Design review of the part built by this model. Coordinates are the model's own, in mm. Face numbers are marked on the shaded views. Give positions to 0.01 mm unless a question says otherwise; leave off trailing zeros. Order: outer loops, then holes, each group sorted by start corner. A loop starts at its lowest first (then second) coordinate and runs counter-clockwise, first axis right, second up.
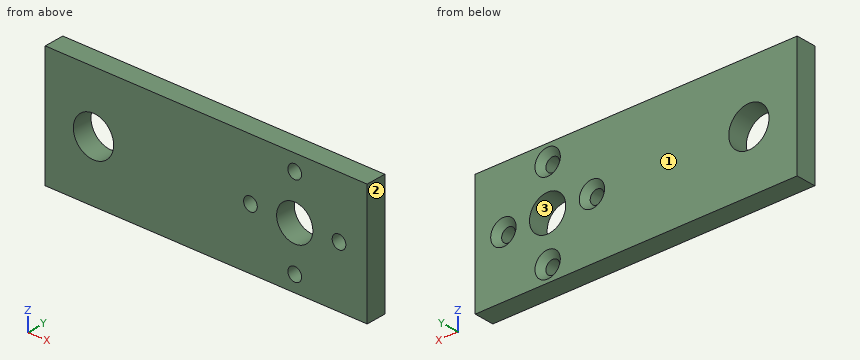
```python
from build123d import *

# Parameters (mm, degrees)
SKETCH1_W                                           = 80
SKETCH1_H                                           = 30
SKETCH1_R                                           = 4.5
SKETCH1_R_2                                         = 5
BOSS_EXTRUDE1_DEPTH                                 = 5
CSK_FOR_M3_COUNTERSUNK_FLAT_HEAD_SCREW1_D           = 3.4
CSK_FOR_M3_COUNTERSUNK_FLAT_HEAD_SCREW1_CSINK_D     = 6.3
CSK_FOR_M3_COUNTERSUNK_FLAT_HEAD_SCREW1_CSINK_ANGLE = 90
CIRPATTERN1_COUNT                                   = 4


with BuildPart() as part:
    # Sketch1 → Boss-Extrude1 (new body)
    with BuildSketch(Plane(origin=(0, 0, 0), x_dir=(1, 0, 0), z_dir=(0, 1, 0))):
        Rectangle(SKETCH1_W, SKETCH1_H)
        with Locations(Location((22, 0, 0), (0, 0, 270))):
            Circle(SKETCH1_R, mode=Mode.SUBTRACT)
        with Locations(Location((-28, 0, 0), (0, 0, 270))):
            Circle(SKETCH1_R_2, mode=Mode.SUBTRACT)
    extrude(amount=BOSS_EXTRUDE1_DEPTH)

    # CSK for M3 Countersunk Flat Head Screw1 (through all)
    with Locations(Plane(origin=(0, 5, 0), x_dir=(1, 0, 0), z_dir=(0, 1, 0))):
        with Locations((11, 0)):
            csk_for_m3_countersunk_flat_head_screw1 = CounterSinkHole(CSK_FOR_M3_COUNTERSUNK_FLAT_HEAD_SCREW1_D / 2, CSK_FOR_M3_COUNTERSUNK_FLAT_HEAD_SCREW1_CSINK_D / 2, counter_sink_angle=CSK_FOR_M3_COUNTERSUNK_FLAT_HEAD_SCREW1_CSINK_ANGLE)

    # CirPattern1: CSK for M3 Countersunk Flat Head Screw1 ×4 about axis
    cirpattern1_axis = Axis((22, 0, 0), (0, 1, 0))
    for i in range(1, CIRPATTERN1_COUNT):
        add(csk_for_m3_countersunk_flat_head_screw1.rotate(cirpattern1_axis, i * 360 / CIRPATTERN1_COUNT), mode=Mode.SUBTRACT)


solid = part.part
```
1. For line 1 along X through (y, z) = (3, 3.75); line 2 along X through (y, z) = (3.05, -1); line 3 along Z through (x, y) = (12, 4.45), list the stretches that pass through material, from the lowest coordinate up.
Recorded:
line 1: x = -40 to -31.31, -24.69 to 19.51, 24.49 to 40
line 2: x = -40 to -32.9, -23.1 to 9.63, 12.37 to 17.61, 26.39 to 31.63, 34.37 to 40
line 3: z = -15 to -2.4, 2.4 to 15
2. For pin 1 (4 mm diameter, centred on x = 22, z = 11, fed in from +Y), flat-tipped, find the tip position at first contact; note if it passes through.
Recorded:
pin 1: stops at y = 3.85
3. Draft analysis for pull direction X (two halves, no side actions). For the marked faces 1, 2 and 3, state which applies: pulls with the +X half, pulls with the -X half, needs draft (parallel to the pull), parting line crosses it, or undercut.
Recorded:
face 1: needs draft
face 2: pulls with the +X half
face 3: undercut
4. Take a section at C-C (x = 22). State the section outline as (y, z) points, then the cut area to 3 significant figures.
Recorded:
outline: (0, -15) - (5, -15) - (5, -14.15) - (3.55, -12.7) - (0, -12.7) - close; (0, -9.3) - (3.55, -9.3) - (5, -7.85) - (5, -4.5) - (0, -4.5) - close; (0, 4.5) - (5, 4.5) - (5, 7.85) - (3.55, 9.3) - (0, 9.3) - close; (0, 12.7) - (3.55, 12.7) - (5, 14.15) - (5, 15) - (0, 15) - close
area: 66.8 mm2
5. Take a section at D-D (x = -28). State the section outline as (y, z) points.
Recorded:
outline: (0, -15) - (5, -15) - (5, -5) - (0, -5) - close; (0, 5) - (5, 5) - (5, 15) - (0, 15) - close
6. Take a section at A-A (z = 0). State the section outline as (x, y) points.
Recorded:
outline: (-40, 0) - (-33, 0) - (-33, 5) - (-40, 5) - close; (-23, 0) - (9.3, 0) - (9.3, 3.55) - (7.85, 5) - (-23, 5) - close; (12.7, 0) - (17.5, 0) - (17.5, 5) - (14.15, 5) - (12.7, 3.55) - close; (26.5, 0) - (31.3, 0) - (31.3, 3.55) - (29.85, 5) - (26.5, 5) - close; (34.7, 0) - (40, 0) - (40, 5) - (36.15, 5) - (34.7, 3.55) - close
7. Take a section at B-B (y = 0.9). State the section outline as (x, z) points.
Recorded:
outline: (-40, -15) - (40, -15) - (40, 15) - (-40, 15) - close; hole circle Ø10 at (-28, 0); hole circle Ø3.4 at (11, 0); hole circle Ø9 at (22, 0); hole circle Ø3.4 at (22, -11); hole circle Ø3.4 at (22, 11); hole circle Ø3.4 at (33, 0)
